Autodesk Inventor part; units mm, degrees
ref_plane "YZ Plane" through (0, 0, 0) normal (1, 0, 0) x (0, 1, 0)
ref_plane "XZ Plane" through (0, 0, 0) normal (0, 1, 0) x (-1, 0, 0)
ref_plane "XY Plane" through (0, 0, 0) normal (0, 0, 1) x (1, 0, 0)
sketch "スケッチ1" plane through (0, 0, 0) normal (0, 0, 1) x (1, 0, 0)
  line L0 (0, 0) -> (-90.3, 0)
  line L1 (-90.3, 0) -> (-90.3, 64.35)
  line L2 (-90.3, 64.35) -> (0, 64.35)
  line L3 (0, 64.35) -> (0, 0)
  line L4 (-90.3, 21.15) -> (0, 21.15)
  line L5 (-55.219, 21.15) -> (-37.813, 0)
  line L6 (-90.3, 29.15) -> (0, 29.15)
  line L7 (-80.3, 29.15) -> (-67.1, 29.15)
  line L8 (-67.1, 29.15) -> (-67.1, 34.35)
  line L9 (-67.1, 34.35) -> (-80.3, 34.35)
  line L10 (-80.3, 34.35) -> (-80.3, 29.15)
  line L11 (-67.1, 29.15) -> (-67.1, 21.15)
  line L12 (-38.44, 64.35) -> (0, 54.9793)
  dimension "d0" = 90.3
  dimension "d1" = 64.35
  dimension "d2" = 21.15
  dimension "d3" = 55.219
  dimension "d4" = 37.813
  dimension "d5" = 35.2
  dimension "d6" = 10
  dimension "d7" = 5.2
  dimension "d8" = 13.2
  dimension "d9" = 166.3
  dimension "d10" = 51.86
extrude "押し出し1" add sketch "スケッチ1" along normal blind 2 contours L0 L5 L4 L3 | L4 L11 L6 L3 | L6 L8 L9 L10 L1 L2 L12 L3
sketch "スケッチ2" plane through (0, 0, 2) normal (0, 0, 1) x (1, 0, 0)
  line L0 (-85.1, 34.75) -> (-53.1, 34.75)
  line L1 (-53.1, 34.75) -> (-53.1, 50.75)
  line L2 (-53.1, 50.75) -> (-85.1, 50.75)
  line L3 (-85.1, 50.75) -> (-85.1, 34.75)
  line L4 (-90.3, 29.15) -> (-80.3, 29.15)
  line L5 (-90.3, 64.35) -> (-90.3, 29.15)
  line L6 (-8.4, 4.75) -> (-24.4, 4.75)
  line L7 (-24.4, 4.75) -> (-24.4, 36.75)
  line L8 (-24.4, 36.75) -> (-8.4, 36.75)
  line L9 (-8.4, 36.75) -> (-8.4, 4.75)
  line L10 (0, 0) -> (0, 54.9793)
  line L11 (-37.813, 0) -> (0, 0)
  dimension "d13" = 5.6
  dimension "d14" = 5.2
  dimension "d15" = 16
  dimension "d16" = 32
  dimension "d17" = 8.4
  dimension "d18" = 4.75
  dimension "d19" = 16
  dimension "d20" = 32
hole "穴1" at (-85.1, 50.75, 2) at (-85.1, 34.75, 2) at (-53.1, 34.75, 2) at (-53.1, 50.75, 2) at (-24.4, 4.75, 2) at (-8.4, 4.75, 2) at (-8.4, 36.75, 2) at (-24.4, 36.75, 2) direction (0, 0, -1) diameter 2.5 end through all
fillet "フィレット1" radius 1 11 edges at (0, 0, 1) (0, 54.9793, 1) (-90.3, 64.35, 1) (-90.3, 29.15, 1) (-80.3, 29.15, 1) (-80.3, 34.35, 1) (-67.1, 34.35, 1) (-67.1, 21.15, 1) (-55.219, 21.15, 1) (-37.813, 0, 1) (-38.44, 64.35, 1)
sketch "スケッチ3" plane through (0, 0, 0) normal (0, 0, -1) x (-1, 0, 0)
  line L0 (31.65, 18.75) -> (39.65, 18.75)
  line L1 (39.65, 18.75) -> (39.65, 32.75)
  line L2 (39.65, 32.75) -> (31.65, 32.75)
  line L3 (31.65, 32.75) -> (31.65, 18.75)
  circle A0 centre (24.4, 4.75) radius 1.25
  circle A1 centre (24.4, 36.75) radius 1.25
  point P0 (0, 0)
  dimension "d29" = 14
  dimension "d30" = 14
  dimension "d31" = 8
  dimension "d32" = 6
extrude "押し出し2" cut sketch "スケッチ3" against normal blind 10 contours L3 L2 L1 L0
fillet "フィレット2" radius 1 4 edges at (-31.65, 18.75, 1) (-31.65, 32.75, 1) (-39.65, 32.75, 1) (-39.65, 18.75, 1)
sketch "スケッチ5" plane through (0, 0, 0) normal (0, 0, -1) x (-1, 0, 0)
  line L0 (79.3, 34.35) -> (68.1, 34.35)
  line L1 (73.3, 34.35) -> (73.3, 64.35)
  line L2 (38.5601, 64.35) -> (89.3, 64.35)
  line L3 (90.3, 63.35) -> (90.3, 30.15)
  arc A0 (80.3, 33.35) -> (79.3, 34.35) centre (79.3, 33.35) ccw
  arc A1 (80.3, 33.35) -> (79.3, 34.35) centre (79.3, 33.35) ccw
  arc A2 (80.3, 30.15) -> (81.3, 29.15) centre (81.3, 30.15) ccw
  arc A3 (80.3, 30.15) -> (81.3, 29.15) centre (81.3, 30.15) ccw
  arc A4 (89.3, 29.15) -> (90.3, 30.15) centre (89.3, 30.15) ccw
  arc A5 (89.3, 29.15) -> (90.3, 30.15) centre (89.3, 30.15) ccw
  arc A6 (90.3, 63.35) -> (89.3, 64.35) centre (89.3, 63.35) ccw
  arc A7 (90.3, 63.35) -> (89.3, 64.35) centre (89.3, 63.35) ccw
  line L4 (73.3, 64.35) -> (89.3, 64.35)
  line L5 (90.3, 63.35) -> (90.3, 30.15)
  line L6 (89.3, 29.15) -> (81.3, 29.15)
  line L7 (80.3, 30.15) -> (80.3, 33.35)
  line L8 (79.3, 34.35) -> (73.3, 34.35)
  point P0 (0, 0)
  dimension "d36" = 17
extrude "押し出し3" cut sketch "スケッチ5" against normal blind 0.19
equation "\"BendRadius\" = Thickness"
equation "\"BendReliefWidth\" = Thickness"
equation "\"BendReliefDepth\" = 0.5 * Thickness"
equation "\"CornerReliefSize\" = 4 * Thickness"
equation "\"MinimumRemnant\" = 2 * Thickness"
equation "\"TransitionRadius\" = BendRadius"
equation "\"JacobiRadiusSize\" = BendRadius"
equation "\"GapSize\" = Thickness"
properties part number "connectplate2" material "アルミニウム 6061"
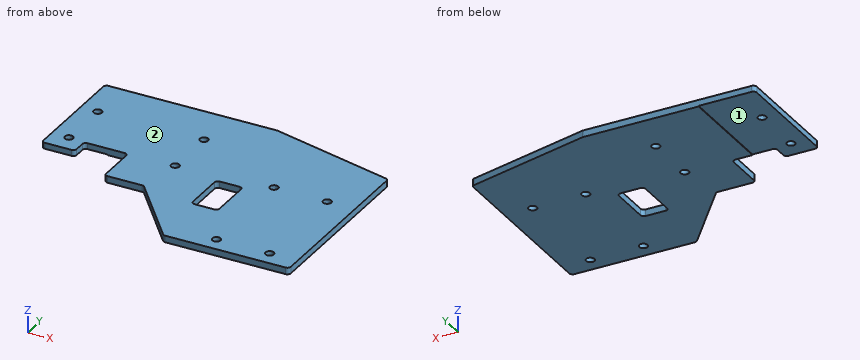
The listing builds one solid part. Answer for the finished solid, in the listing's coordinates (mm). Face numbers are marked on the shaded views. A direction names the side the tool comes from. Give positions to 0.01 mm unless a question says otherwise; leave off trailing zeros. Order: outer loops, then holes, each group sorted by start corner. A loop starts at its lowest first (then second) coordinate and runs counter-clockwise, first axis right, second up.
Item 1: Which of the six approach directions +Z, -Z, +X, -X, +Y, -Y give full straight-line access (tool end or side, diameter ignored) to the marked faces 1 and 2?
From the geometry:
face 1: -Z, -X, +Y, -Y
face 2: +Z, +X, -X, +Y, -Y
Item 2: Given pin 1 Ø2 at (x, y) = (-85.1, 50.75) entering from +Z; pin 2 Ø0.6 at (y, z) = (26, 1) entering from -X; pin 3 Ø1 at (x, z) = (-61.5, 1) entering from -Y, each flat-ended and moving along its own axis, determine where each tip first touches the part or whether it passes through.
From the geometry:
pin 1: passes through
pin 2: stops at x = -67.1
pin 3: stops at y = 21.15
Item 3: The part is cut by section B-B, the plane x = -85.1. Give the vertices of the cut face in (y, z), and give its area (3 significant figures).
From the geometry:
outline: (29.15, 0.19) - (33.5, 0.19) - (33.5, 2) - (29.15, 2) - close; (36, 0.19) - (49.5, 0.19) - (49.5, 2) - (36, 2) - close; (52, 0.19) - (64.35, 0.19) - (64.35, 2) - (52, 2) - close
area: 54.7 mm2
Item 4: The part is cut by section D-D, the plane x = -8.4. Give the vertices of the cut face in (y, z).
From the geometry:
outline: (0, 0) - (3.5, 0) - (3.5, 2) - (0, 2) - close; (6, 0) - (35.5, 0) - (35.5, 2) - (6, 2) - close; (38, 0) - (57.03, 0) - (57.03, 2) - (38, 2) - close
Item 5: The part is cut by section C-C, the plane z = 1.7. Count the separate pieces of the cut face and the enclosed holes in it, and give its area (3 significant figures).
From the geometry:
separate pieces: 1
enclosed holes: 9
area: 4,300 mm2
Item 6: Find the intervals of material crossed by probe 1 along X at (y, z) = (30.5, 0.9); probe 2 along X at (y, z) = (34.75, 0.95); probe 3 along X at (y, z) = (28, 0.35), in increasing order.
From the geometry:
probe 1: x = -90.3 to -80.3, -67.1 to -39.65, -31.65 to 0
probe 2: x = -90.3 to -86.35, -83.85 to -54.35, -51.85 to 0
probe 3: x = -67.1 to -39.65, -31.65 to 0
Item 7: The part is cut by section A-A, the plane y = 23.5. Give the vertices of the cut face in (x, z), and give its area (3 significant figures).
From the geometry:
outline: (-67.1, 0) - (-39.65, 0) - (-39.65, 2) - (-67.1, 2) - close; (-31.65, 0) - (0, 0) - (0, 2) - (-31.65, 2) - close
area: 118 mm2
